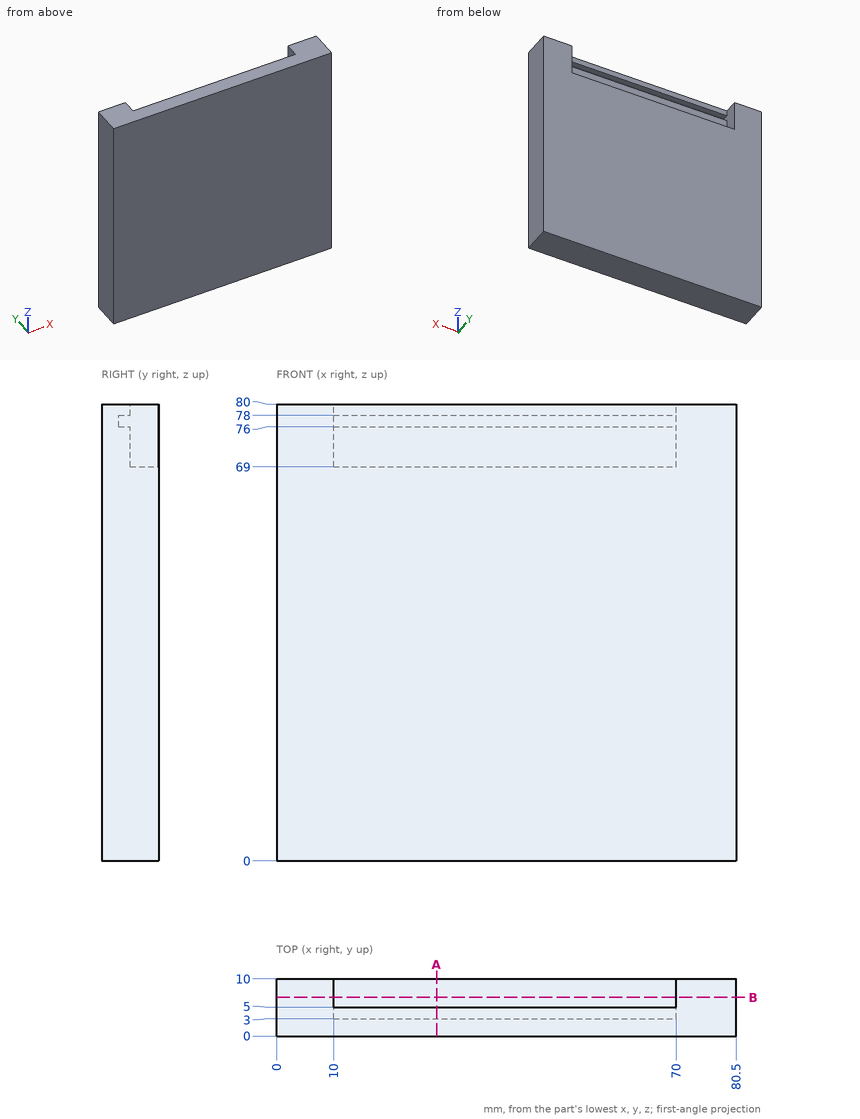
Part print with two shaded views. Sizes in mm from the minimum x, y, z corner. Coordinates: 2 decimals unless noted, no trailing zeros. Write each loop counter-clockwise with the first axis right and the second up, starting at its lowest first coordinate (ties: lowest second). Pieces come first, ordered by that corner, then holes.
(1) Drill centre lines: line 1 (Z direction, x = 35, y = 4); line 2 (Z direction, x = 52.5, y = 9.75); line 3 (Y direction, x = 30.5, z = 72). Where is each one in solid material? Low to high.
(2) Cut at B-B on y = 6.75. List the corners of the cut face in (x, z), and give its area (3 significant figures).
(3) Cut at A-A on x = 28. List the corners of the cut face in (y, z).
(4) Pin check, flat tips, straight feed: pin 1 Ø2 at (x, z) = (45, 79) entering from +Y; pin 2 Ø1 at (y, z) = (4, 18) entering from -X. Stop position of each tip, or through.
Working result:
1. line 1: z = 0 to 76, 78 to 80
1. line 2: z = 0 to 69
1. line 3: y = 0 to 5
2. outline: (0, 0) - (80.5, 0) - (80.5, 80) - (70, 80) - (70, 69) - (10, 69) - (10, 80) - (0, 80) - close
2. area: 5,780 mm2
3. outline: (0, 0) - (10, 0) - (10, 69) - (5, 69) - (5, 76) - (3, 76) - (3, 78) - (5, 78) - (5, 80) - (0, 80) - close
4. pin 1: stops at y = 5
4. pin 2: stops at x = 0
